Here's the drawing with two shaded views (mm, measured from the low corner). I have some questions. A direction names the side the tool comes from. Give positions to 0.01 mm unless a question says otherwise; leave off trailing zeros. Loops run counter-clockwise (first coordinate to the right, second up) from the corner with the lowest first, then second, coordinate; pieces in that order, holes last. Notation, with made-up numbers: (64.25, -35.5) -> (93.25, -35.5) arc R29 ccw to (93.25, 3.5) -> close; hole circle Ø1 at (-32, 23.25). An arc over 180 degrees is marked (long way). Answer in a Markdown table with one row per item. Add a question column.
Item 1: Which directions (+Z, -Z, +X, -X, +Y, -Y) give clear straight access to the entire face, cutting with the end or side of a thin tool? Please do the marked faces 4, 5 and 6.
Item 2: If we section it at B-B (x = 14): Write out the boundary of the cut face in (y, z), then the cut area to 3 significant figures.
Item 3: If we section it at C-C (z = 17.5): Write out the boundary of the cut face in (x, y), then the cut area to 3 significant figures.
Item 4: If I drill on line 1 (Z direction, x = 14, y = 10.3); line 2 (Y direction, x = 24, z = 1.6); line 3 (Y direction, x = 13, z = 5), over which ranges is the centre line in solid material (lowest first)?
Item 5: If we section it at A-A (y = 10): Write out the boundary of the cut face in (x, z).
Item 6: For P1, Ø1.5, axis at y = 9.5, z = 8, coming from the -X side; P2, Ø6, axis at x = 22, z = 7.5, coming from the +Y side; P3, Ø5, axis at x = 24, y = 3.5, coming from the +Z side, each with a flat end and sliding along its axis, tell me the tip position at first contact or that it passes through.
Item 7: We'd pull the mould along X, two halves only. Please class the marked faces 1, 2 and 3: released by +X, released by -X, zero draft, split by the parting line, or undercut.
Item 8: If we section it at D-D (x = 24): Write out the boundary of the cut face in (y, z).
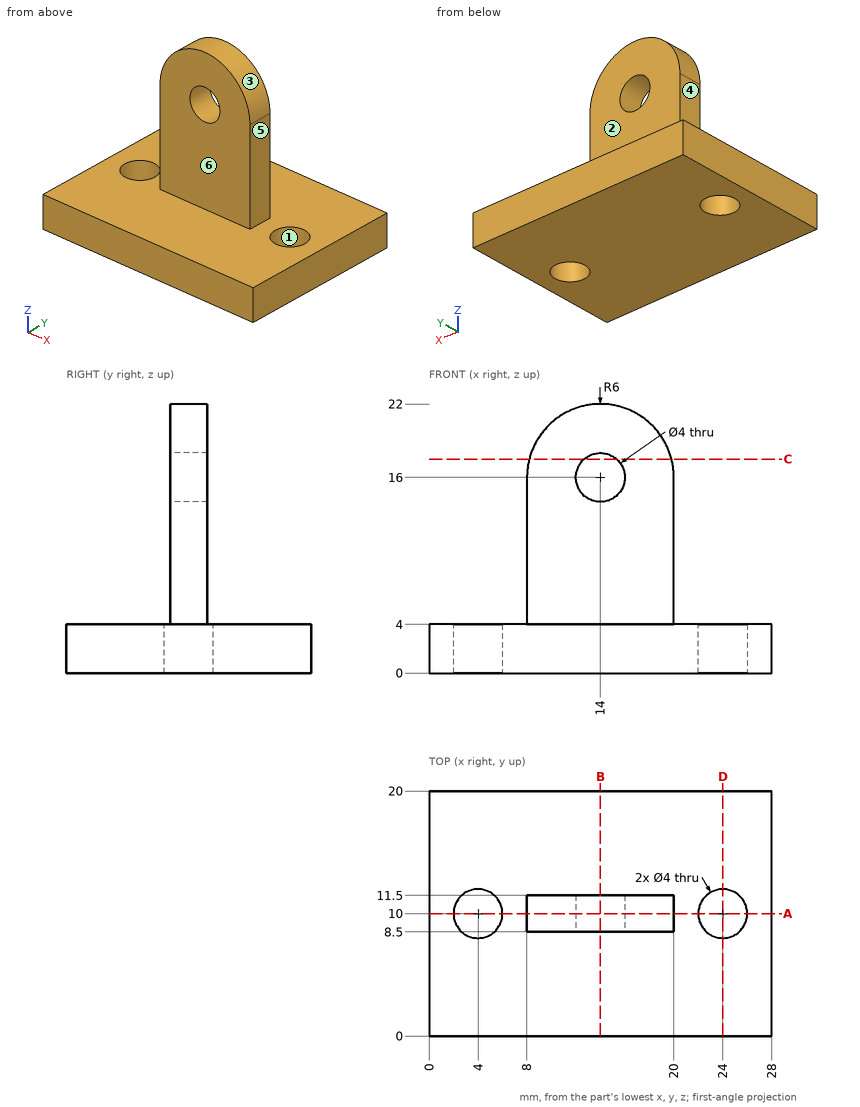
Recorded:
| question | item | result |
|---|---|---|
| 1 | face 4 | +Z, -X, +Y, -Y |
| 1 | face 5 | +Z, +X, +Y, -Y |
| 1 | face 6 | +Z, +X, -X, -Y |
| 2 | outline | (0, 0) -> (20, 0) -> (20, 4) -> (11.5, 4) -> (11.5, 14) -> (8.5, 14) -> (8.5, 4) -> (0, 4) -> close; (8.5, 18) -> (11.5, 18) -> (11.5, 22) -> (8.5, 22) -> close |
| 2 | area | 122 mm^2 |
| 3 | outline | (8.19, 8.5) -> (12.68, 8.5) -> (12.68, 11.5) -> (8.19, 11.5) -> close; (15.32, 8.5) -> (19.81, 8.5) -> (19.81, 11.5) -> (15.32, 11.5) -> close |
| 3 | area | 26.9 mm^2 |
| 4 | line 1 | z = 0 to 14, 18 to 22 |
| 4 | line 2 | y = 0 to 8, 12 to 20 |
| 4 | line 3 | y = 8.5 to 11.5 |
| 5 | outline | (0, 0) -> (2, 0) -> (2, 4) -> (0, 4) -> close; (6, 0) -> (22, 0) -> (22, 4) -> (20, 4) -> (20, 16) arc R6 ccw to (8, 16) -> (8, 4) -> (6, 4) -> close; (26, 0) -> (28, 0) -> (28, 4) -> (26, 4) -> close; hole circle Ø4 at (14, 16) |
| 6 | P1 | stops at x = 8 |
| 6 | P2 | stops at y = 11.5 |
| 6 | P3 | stops at z = 4 |
| 7 | face 1 | undercut |
| 7 | face 2 | zero draft |
| 7 | face 3 | split by the parting line |
| 8 | outline | (0, 0) -> (8, 0) -> (8, 4) -> (0, 4) -> close; (12, 0) -> (20, 0) -> (20, 4) -> (12, 4) -> close |
